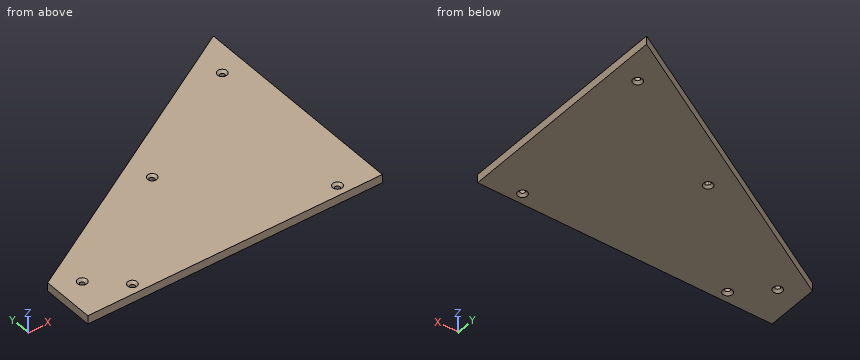
```python
from build123d import *

# Parameters (mm, degrees)
RESSALTO_EXTRUS_O3_DEPTH                       = 8
ESCAREADO_PARA_SFHCS_M42_D                     = 4.5
ESCAREADO_PARA_SFHCS_M42_CSINK_D               = 8.96
ESCAREADO_PARA_SFHCS_M42_CSINK_ANGLE           = 90
RESSALTO_EXTRUS_O5_DEPTH                       = 8
ESCAREADO_PARA_SFHCS_M44_D                     = 4.5
ESCAREADO_PARA_SFHCS_M44_CSINK_D               = 8.96
ESCAREADO_PARA_SFHCS_M44_CSINK_ANGLE           = 90
ESCAREADO_PARA_SFHCS_M46_D                     = 4.5
ESCAREADO_PARA_SFHCS_M46_CSINK_D               = 8.96
ESCAREADO_PARA_SFHCS_M46_CSINK_ANGLE           = 90
ESCAREADO_PARA_SFHCS_M47_D                     = 4.5
ESCAREADO_PARA_SFHCS_M47_CSINK_D               = 8.96
ESCAREADO_PARA_SFHCS_M47_CSINK_ANGLE           = 90
ESCAREADO_PARA_SFHCS_M47_ON_FACE_2_D           = 4.5
ESCAREADO_PARA_SFHCS_M47_ON_FACE_2_CSINK_D     = 8.96
ESCAREADO_PARA_SFHCS_M47_ON_FACE_2_CSINK_ANGLE = 90


# Read off the part's stored shape, not the designer's step: Escareado para SFHCS M45
with BuildPart() as part:
    # Esboço1 → Ressalto-extrusão3 (new body)
    with BuildSketch(Plane.XY):
        Polygon((0, 20), (280, 170), (0, 0), align=None)
        Polygon((280, 0), (280, 170), (0, 0), align=None)
    extrude(amount=RESSALTO_EXTRUS_O3_DEPTH)

    # Escareado para SFHCS M42 (through all)
    with Locations(Plane(origin=(50, 10, 8), x_dir=(1, 0, 0), z_dir=(0, 0, 1))):
        with Locations((0, 0), (195, 0)):
            CounterSinkHole(ESCAREADO_PARA_SFHCS_M42_D / 2, ESCAREADO_PARA_SFHCS_M42_CSINK_D / 2, counter_sink_angle=ESCAREADO_PARA_SFHCS_M42_CSINK_ANGLE)

    # Esboço6 → Ressalto-extrusão5 (add, through all)
    with BuildSketch(Plane.XY.offset(8)):
        Polygon((0, 20), (0, 50), (280, 210), (280, 170), align=None)
    extrude(amount=-RESSALTO_EXTRUS_O5_DEPTH)

    # Escareado para SFHCS M44 (through all)
    with Locations(Plane(origin=(21.706078553, 35.403473459, 8), x_dir=(1, 0, 0), z_dir=(0, 0, 1))):
        with Locations((0, 0), (236.587842894, 135.193053082)):
            CounterSinkHole(ESCAREADO_PARA_SFHCS_M44_D / 2, ESCAREADO_PARA_SFHCS_M44_CSINK_D / 2, counter_sink_angle=ESCAREADO_PARA_SFHCS_M44_CSINK_ANGLE)

    # Escareado para SFHCS M45 outline → Escareado para SFHCS M45 (revolve, cut)
    with BuildSketch(Plane(origin=(245, 10, 0), x_dir=(1, 0, 0), z_dir=(0, -1, 0))):
        Polygon((4.48, 0), (2.25, 2.23), (2.25, 0), align=None)
    revolve(axis=Axis((245, 10, 0), (0, 0, 1)), mode=Mode.SUBTRACT)

    # Escareado para SFHCS M46 (through all)
    with Locations(Plane(origin=(258.293921447, 170.596526541, 0), x_dir=(-1, 0, 0), z_dir=(0, 0, -1))):
        with Locations((0, 0), (236.587842894, -135.193053082), (208.293921447, -160.596526541)):
            CounterSinkHole(ESCAREADO_PARA_SFHCS_M46_D / 2, ESCAREADO_PARA_SFHCS_M46_CSINK_D / 2, counter_sink_angle=ESCAREADO_PARA_SFHCS_M46_CSINK_ANGLE)

    # Escareado para SFHCS M47 (through all)
    with Locations(Plane(origin=(140, 103, 8), x_dir=(1, 0, 0), z_dir=(0, 0, 1))):
        with Locations((0, 0)):
            CounterSinkHole(ESCAREADO_PARA_SFHCS_M47_D / 2, ESCAREADO_PARA_SFHCS_M47_CSINK_D / 2, counter_sink_angle=ESCAREADO_PARA_SFHCS_M47_CSINK_ANGLE)

    # Escareado para SFHCS M47 on face 2 (through all)
    with Locations(Plane(origin=(139.792651332, 103.260866722, 0), x_dir=(-1, 0, 0), z_dir=(0, 0, -1))):
        with Locations((0, 0)):
            CounterSinkHole(ESCAREADO_PARA_SFHCS_M47_ON_FACE_2_D / 2, ESCAREADO_PARA_SFHCS_M47_ON_FACE_2_CSINK_D / 2, counter_sink_angle=ESCAREADO_PARA_SFHCS_M47_ON_FACE_2_CSINK_ANGLE)


solid = part.part
```
CAD build for the part. Positions are in the model's coordinates, mm. Coordinates: 2 decimals unless noted, no trailing zeros. Order: outer loops, then holes, each group sorted by start corner. A loop starts at its lowest first (then second) coordinate and runs counter-clockwise, first axis right, second up. Notation, with made-up numbers: (47.25, 48) - (88.25, 48) arc R30 ccw to (88.25, 84) - close; hole circle Ø2 at (-34, -36.5). An arc over 180 degrees is marked (long way). Answer in a Markdown table with one row per item.
1. Drill centre lines: L1, parallel to X at y = 10, z = 3.95; L2, parallel to Y at x = 48.5, z = 4; L3, parallel to Y at x = 48, z = 4.25. Where is each one in solid material? Low to high. Write a range as from..to.
Answer:
| item | result |
|---|---|
| L1 | 0..47.75, 52.25..242.75, 247.25..280 |
| L2 | 0..8.32, 11.68..77.71 |
| L3 | 0..8.97, 11.03..77.43 |
2. Flat gauge pins, fed straight in: P1, Ø4, axis at y = 132.5, z = 4.5, coming from the -X side (3 decimals); P2, Ø5, axis at x = 258.29, y = 170.6, coming from the -Z side; P3, Ø3, axis at x = 143, z = 6, coming from the +Y side. Where does each tip first touch, or does it go through?
Answer:
| item | result |
|---|---|
| P1 | x = 140.875 |
| P2 | z = 1.97 |
| P3 | y = 132.57 |
3. Slice it at B-B, the plane y = 145. List the corners of the cut face in (x, z), then the cut area to 3 significant figures.
Answer:
| item | result |
|---|---|
| outline | (166.25, 0) - (280, 0) - (280, 8) - (166.25, 8) - close |
| area | 910 mm² |
4. Slice it at A-A, the plane x = 119. List the corners of the cut face in (y, z).
Answer:
| item | result |
|---|---|
| outline | (0, 0) - (118, 0) - (118, 8) - (0, 8) - close |
